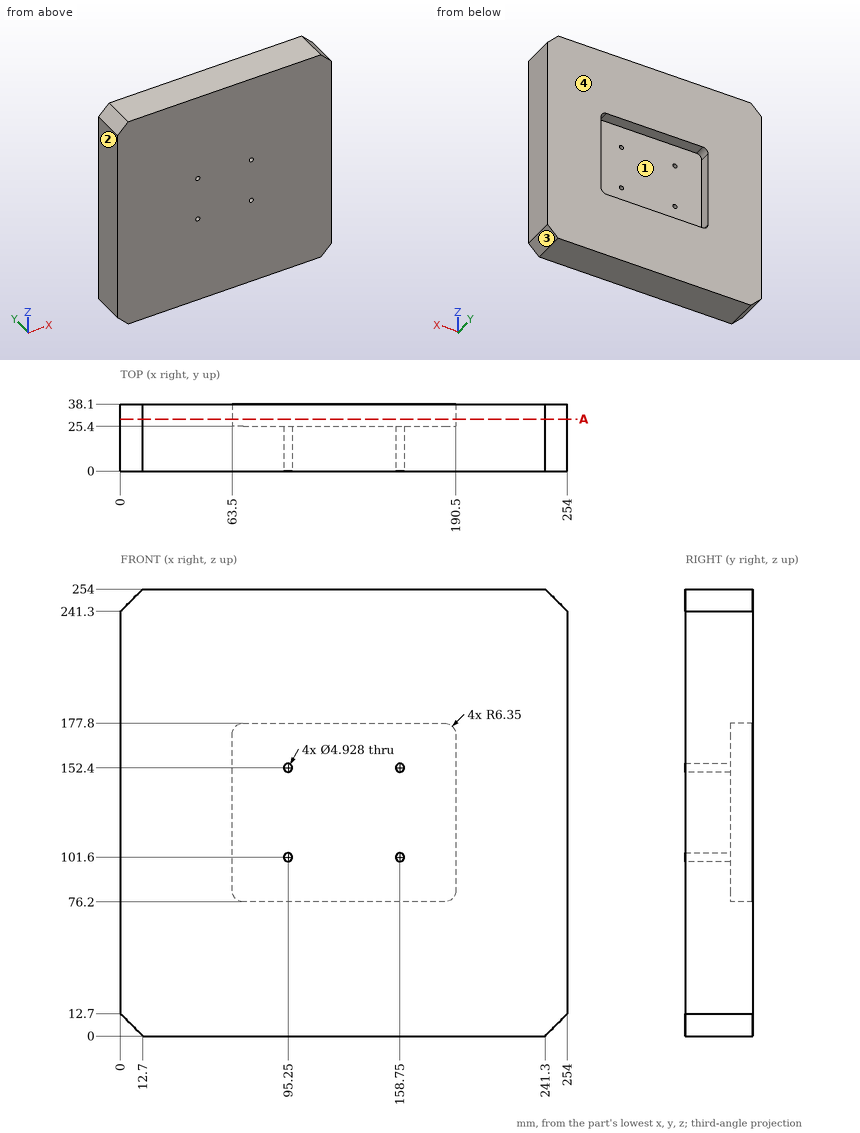
Print and shaded views of the part. All mm, measured from the part's lowest x, y and z. Round coordinates to 2 decimals unless told otherwise and drop trailing zeros. Write each loop counter-clockwise with the first axis right and the second up, starting at its lowest first coordinate (ties: lowest second). Pieces come first, ordered by that corner, then holes. Notation, with made-up numbers: M 69,-5.5 L 121,-5.5 A15 cw 121,15.5 Z; hole C 20.5,-35 d4. An arc over 180 degrees is marked long. Use a Markdown table: item, result. Add a question column.
1. Pull direction X, two halves, no side cores. Call the marked faces 1, 2, 3 and 4: released by +X, released by -X, zero draft, split by the parting line, or undercut.
2. Slice it at A-A on y = 29.5. Give the cut face in (x, z).
3. Drill centre lines: probe 1 along X at (y, z) = (11.5, 152.4); probe 2 along Z at (x, y) = (95.25, 10); probe 3 along Z at (x, y) = (158, 15). Where is each one in solid material? Low to high.
4. Flat gauge pin, fed straight in: P1, Ø5.5, axis at x = 158.75, z = 152.4, coming from the -Y side. Where does the tip first touch, or does it go through?
Reply:
| question | item | result |
|---|---|---|
| 1 | face 1 | undercut |
| 1 | face 2 | released by -X |
| 1 | face 3 | released by +X |
| 1 | face 4 | zero draft |
| 2 | outline | M 0,12.7 L 12.7,0 L 241.3,0 L 254,12.7 L 254,241.3 L 241.3,254 L 12.7,254 L 0,241.3 Z; hole M 63.5,82.55 A6.35 ccw 69.85,76.2 L 184.15,76.2 A6.35 ccw 190.5,82.55 L 190.5,171.45 A6.35 ccw 184.15,177.8 L 69.85,177.8 A6.35 ccw 63.5,171.45 Z |
| 3 | probe 1 | x = 0 to 92.79, 97.71 to 156.29, 161.21 to 254 |
| 3 | probe 2 | z = 0 to 99.14, 104.06 to 149.94, 154.86 to 254 |
| 3 | probe 3 | z = 0 to 99.25, 103.95 to 150.05, 154.75 to 254 |
| 4 | P1 | stops at y = 0 |
